Could you check a few things on this model? Use its own coordinates, in mm. A direction names the side the tool comes from. Round coordinates to 2 decimals unless told otherwise and drop trailing zeros. Loops run counter-clockwise (first coordinate to the right, second up) from the corner with the lowest first, then second, coordinate; pieces in that order, holes last. Notation, with made-up numbers: (7, 1) -> (28, 1) arc R32 cw to (28, 39) -> close; hole circle Ø4 at (-31, -39). An arc over 180 degrees is marked (long way). Write each question's results on one line, items separated by ' | '. Start each with the question number.
1) Imagine slicing it at C-C, the plane y = 1.5. List the corners of the cut face in (x, z) for me.
2) For P1, Ø1.5, axis at x = -14.5, y = 6, coming from the -Z side; P2, Ø3, axis at x = 2.5, y = 2, coming from the -Z side; P3, Ø0.8, axis at x = 13, z = 9, coming from the +Y side, each with a flat end and sliding along its axis, tell me the tip position at first contact or that it passes through.
3) We'd pull the mould along X, two halves only. Please class faces 1 (the flat face through (0, 6, 2.5)), 2 (the flat face through (-20, 3, 0)), 3 (the flat face through (0, 7, 0.254)): pulls with the +X half, pulls with the -X half, needs draft (parallel to the pull), parting line crosses it, or undercut.
4) Imagine slicing it at A-A, the plane y = 7.5. List the corners of the cut face in (x, z) for me.
5) If I drill on probe 1 along Z at (x, y) = (17, 8.5); probe 2 along X at (y, z) = (2.25, 4.75); probe 3 along Z at (x, y) = (16, 6), over which ranges is the centre line in solid material (lowest first)?
6) Which directions (+Z, -Z, +X, -X, +Y, -Y) give clear straight access to the entire face, cutting with the end or side of a thin tool? Please do faces 4 (the flat face through (15, 2, 9)), 5 (the flat face through (0, 7, -0.254)), 6 (the flat face through (15, 2, -9)).
7) Imagine slicing it at B-B, the plane x = 1. List the corners of the cut face in (y, z) for me.
from build123d import *

# Parameters (mm, degrees)
ESQUISSE1_W             = 40
ESQUISSE1_H             = 5
BOSS_EXTRU_1_DEPTH      = 10
ESQUISSE2_W             = 40
ESQUISSE2_H             = 0.508359338
ENL_V_MAT_EXTRU_1_DEPTH = 6
BOSS_EXTRU_2_START      = -12
ESQUISSE3_W             = 10
ESQUISSE3_H             = 2
BOSS_EXTRU_2_DEPTH      = 19
CONG_1_SIZE             = 6
CONG_1_SIZE_2           = 5
CONG_2_SIZE             = 6
CONG_2_SIZE_2           = 5
CONG_4_SIZE             = 6
CONG_4_SIZE_2           = 5
CONG_5_SIZE             = 6
CONG_5_SIZE_2           = 5


with BuildPart() as part:
    # Esquisse1 → Boss.-Extru.1 (new body)
    with BuildSketch(Plane(origin=(0, 0, 0), x_dir=(1, 0, 0), z_dir=(0, 1, 0))):
        Rectangle(ESQUISSE1_W, ESQUISSE1_H)
    extrude(amount=BOSS_EXTRU_1_DEPTH)

    # Esquisse2 → Enlèv. mat.-Extru.1 (cut)
    with BuildSketch(Plane(origin=(0, 10, 0), x_dir=(1, 0, 0), z_dir=(0, 1, 0))):
        Rectangle(ESQUISSE2_W, ESQUISSE2_H)
    extrude(amount=-ENL_V_MAT_EXTRU_1_DEPTH, mode=Mode.SUBTRACT)

    # Esquisse3 → Boss.-Extru.2 (add)
    with BuildSketch(Plane.XY.offset(2.5).offset(BOSS_EXTRU_2_START)):
        with Locations((-15, 1)):
            Rectangle(ESQUISSE3_W, ESQUISSE3_H)
    boss_extru_2 = extrude(amount=BOSS_EXTRU_2_DEPTH)

    # Symétrie1: Boss.-Extru.2 across plane
    add(boss_extru_2.mirror(Plane(origin=(0, 0, 0), x_dir=(0, 0, 1), z_dir=(1, 0, 0))))

    # Congé1
    # an asymmetric fillet: 6, 5 mm, written as the material it adds along each edge
    with BuildSketch(Plane(origin=(-20, 2, 2.5), x_dir=(0, 0, 1), z_dir=(1, 0, 0))) as cong_1_piece_1:
        with BuildLine():
            Bezier((CONG_1_SIZE, 0), (0, 0), (0, -CONG_1_SIZE_2), weights=[1, 0.707106781, 1])
            Line((0, -CONG_1_SIZE_2), (0, 0))
            Line((0, 0), (CONG_1_SIZE, 0))
        make_face()
    extrude(amount=10)

    # Congé2
    # an asymmetric fillet: 6, 5 mm, written as the material it adds along each edge
    with BuildSketch(Plane(origin=(20, 2, 2.5), x_dir=(0, 0, 1), z_dir=(-1, 0, 0))) as cong_2_piece_1:
        with BuildLine():
            Bezier((CONG_2_SIZE, 0), (0, 0), (0, CONG_2_SIZE_2), weights=[1, 0.707106781, 1])
            Line((0, CONG_2_SIZE_2), (0, 0))
            Line((0, 0), (CONG_2_SIZE, 0))
        make_face()
    extrude(amount=10)

    # Congé4
    # an asymmetric fillet: 6, 5 mm, written as the material it adds along each edge
    with BuildSketch(Plane(origin=(10, 2, -2.5), x_dir=(0, 0, -1), z_dir=(1, 0, 0))) as cong_4_piece_1:
        with BuildLine():
            Bezier((CONG_4_SIZE, 0), (0, 0), (0, CONG_4_SIZE_2), weights=[1, 0.707106781, 1])
            Line((0, CONG_4_SIZE_2), (0, 0))
            Line((0, 0), (CONG_4_SIZE, 0))
        make_face()
    extrude(amount=10)

    # Congé5
    # an asymmetric fillet: 6, 5 mm, written as the material it adds along each edge
    with BuildSketch(Plane(origin=(-10, 2, -2.5), x_dir=(0, 0, -1), z_dir=(-1, 0, 0))) as cong_5_piece_1:
        with BuildLine():
            Bezier((CONG_5_SIZE, 0), (0, 0), (0, -CONG_5_SIZE_2), weights=[1, 0.707106781, 1])
            Line((0, -CONG_5_SIZE_2), (0, 0))
            Line((0, 0), (CONG_5_SIZE, 0))
        make_face()
    extrude(amount=10)


solid = part.part
Checked values:
1) outline: (-20, -9.5) -> (-10, -9.5) -> (-10, -2.5) -> (10, -2.5) -> (10, -9.5) -> (20, -9.5) -> (20, 9.5) -> (10, 9.5) -> (10, 2.5) -> (-10, 2.5) -> (-10, 9.5) -> (-20, 9.5) -> close
2) P1: z = -2.88 | P2: z = -2.5 | P3: y = 2
3) face 1: undercut | face 2: pulls with the -X half | face 3: needs draft
4) outline: (-20, -2.5) -> (20, -2.5) -> (20, -0.25) -> (-20, -0.25) -> close; (-20, 0.25) -> (20, 0.25) -> (20, 2.5) -> (-20, 2.5) -> close
5) probe 1: -2.5 to -0.25, 0.25 to 2.5 | probe 2: -20 to -10, 10 to 20 | probe 3: -2.62 to -0.25, 0.25 to 2.62
6) face 4: +Z, +X, -X, +Y | face 5: +X, -X, +Y | face 6: -Z, +X, -X, +Y
7) outline: (0, -2.5) -> (10, -2.5) -> (10, -0.25) -> (4, -0.25) -> (4, 0.25) -> (10, 0.25) -> (10, 2.5) -> (0, 2.5) -> close
